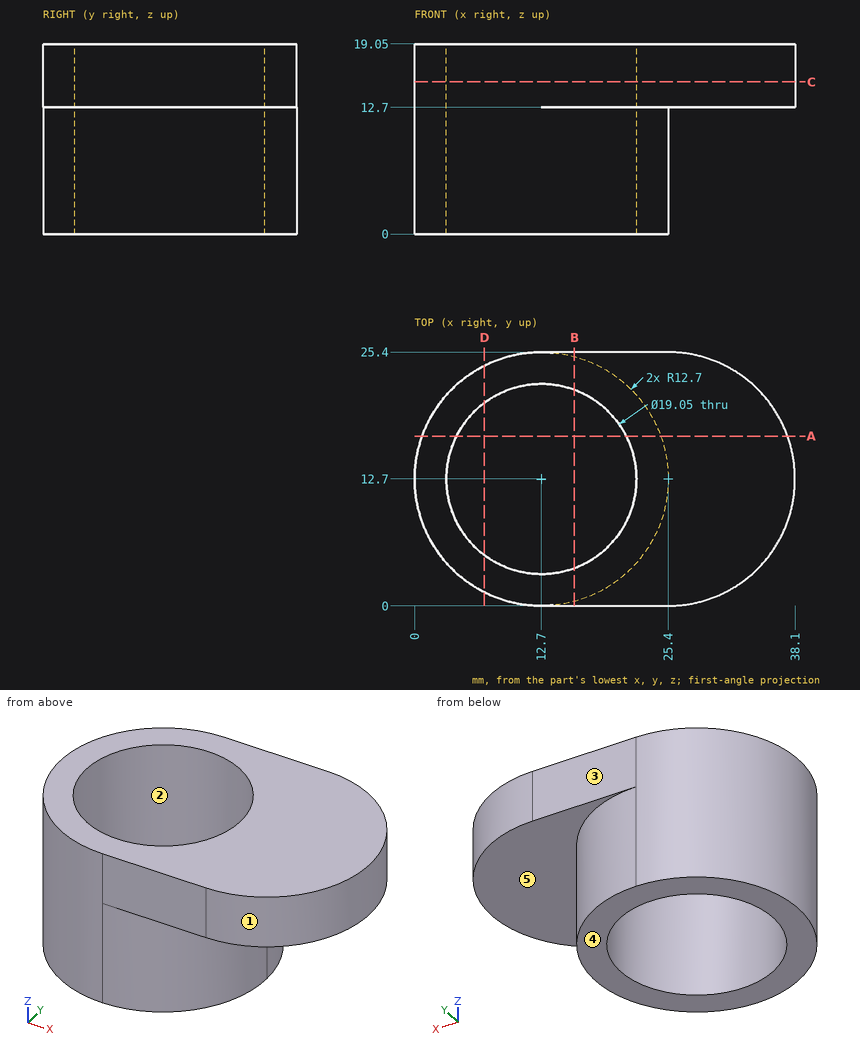
The figure shows three views and two pictorial views of one solid part (mm, origin at its lowest corner). Answer the questions. A direction names the side the tool comes from. Give positions to 0.01 mm unless a question says otherwise; leave off trailing zeros. Order: outer loops, then holes, each group sorted by start corner. A loop starts at its lowest first (then second) coordinate and runs counter-clockwise, first axis right, second up. Notation, with made-up numbers: (56.5, 10) -> (114.5, 10) arc R35 ccw to (114.5, 49) -> close; hole circle Ø3 at (70.5, -2). An arc over 180 degrees is marked (long way). Answer as a JSON object with one key per item and string values. Group by question number.
Item 1: The part is cut by section D-D on x = 7. Write down the section's boundary in (y, z), and give its area (3 significant figures).
Item 2: The part is cut by section B-B on x = 16. Write down the section's boundary in (y, z), and give its area (3 significant figures).
Item 3: Flat-ended cylindrical pins translate along their axes: pin 1 (1.5 mm diameter, centred on y = 19.5, z = 2.5, fed in from -X); pin 2 (6 mm diameter, centred on x = 23, y = 10.5, fed in from -Z); pin 3 (8 mm diameter, centred on y = 19, z = 13.5, fed in from -X); pin 4 (1 mm diameter, centred on x = 16.5, z = 8, fed in from +Y). Find the tip coordinate at first contact, or state that the pin passes through.
Item 4: The part is cut by section C-C on z = 15.25. Write down the section's boundary in (x, y) (3 decimals).
Item 5: The part is cut by section A-A on y = 17. Write down the section's boundary in (x, z), and give its area (3 significant figures).
Item 6: Determine the mould class of the marked faces 1, 2 and 3 for opening direction X: pulls with the +X half, pulls with the -X half, needs draft (parallel to the pull), parting line crosses it, or undercut.
Item 7: A tool of negligible diameter and unlimited length cuts with its end or side. For the marked faces 4 and 5, from which of +Z, -Z, +X, -X, +Y, -Y can it reach the whole face along a straight path? Write none if from no direction.
Item 8: Consider L1, parallel to X at y = 12.7, z = 14.5 (3 decimals); L2, parallel to X at y = 12.7, z = 11.75 (3 decimals). Determine where each line is inside the solid, lowest interval first. Write a range as from..to.
Result set:
{
 "1": {"outline": "(1.35, 0) -> (5.07, 0) -> (5.07, 19.05) -> (1.35, 19.05) -> close; (20.33, 0) -> (24.05, 0) -> (24.05, 19.05) -> (20.33, 19.05) -> close", "area": "142 mm²"},
 "2": {"outline": "(0, 12.7) -> (0.44, 12.7) -> (0.44, 0) -> (3.76, 0) -> (3.76, 19.05) -> (0, 19.05) -> close; (21.64, 0) -> (24.96, 0) -> (24.96, 12.7) -> (25.4, 12.7) -> (25.4, 19.05) -> (21.64, 19.05) -> close", "area": "132 mm²"},
 "3": {"pin 1": "x = 1.53", "pin 2": "z = 0", "pin 3": "x = 0.21", "pin 4": "y = 24.96"},
 "4": {"outline": "(12.7, 0) -> (25.4, 0) arc R12.7 ccw to (25.4, 25.4) -> (12.7, 25.4) arc R12.7 ccw to start; hole circle Ø19.05 at (12.7, 12.7)"},
 "5": {"outline": "(0.75, 0) -> (4.2, 0) -> (4.2, 19.05) -> (0.75, 19.05) -> close; (21.2, 0) -> (24.65, 0) -> (24.65, 12.7) -> (37.35, 12.7) -> (37.35, 19.05) -> (21.2, 19.05) -> close", "area": "212 mm²"},
 "6": {"face 1": "pulls with the +X half", "face 2": "undercut", "face 3": "needs draft"},
 "7": {"face 4": "-Z, +X, -X, +Y, -Y", "face 5": "-Z, +X"},
 "8": {"L1": "0..3.175, 22.225..38.1", "L2": "0..3.175, 22.225..25.4"}
}
